```python
from build123d import *

# Parameters (mm, degrees)
BOSS_EXTRUDE1_DEPTH      = 80
F_6_0_6_DIAMETER_HOLE1_D = 6
F_8_0_8_DIAMETER_HOLE1_D = 8
F_6_0_6_DIAMETER_HOLE2_D = 6


with BuildPart() as part:
    # Sketch2 → Boss-Extrude1 (new body)
    with BuildSketch(Plane.XY):
        Polygon((0, 0), (31.153008197, 0), (31.153008197, 120), (0, 120), (0, 110.293748295), (20, 110.293748295), (20, 9.706251705), (0, 9.706251705), align=None)
    extrude(amount=BOSS_EXTRUDE1_DEPTH)

    # Ø6.0 (6) Diameter Hole1 (through all)
    with Locations(Plane(origin=(0, 120, 0), x_dir=(1, 0, 0), z_dir=(0, 1, 0))):
        with Locations((10, -15)):
            Hole(F_6_0_6_DIAMETER_HOLE1_D / 2)

    # Ø8.0 (8) Diameter Hole1 (through all)
    with Locations(Plane(origin=(31.153008197, 0, 0), x_dir=(0, 0, -1), z_dir=(1, 0, 0))):
        with Locations((-45, 30)):
            Hole(F_8_0_8_DIAMETER_HOLE1_D / 2)

    # Ø6.0 (6) Diameter Hole2 (through all)
    with Locations(Plane(origin=(0, 120, 0), x_dir=(1, 0, 0), z_dir=(0, 1, 0))):
        with Locations((11.153008197, -65)):
            Hole(F_6_0_6_DIAMETER_HOLE2_D / 2)


solid = part.part
```
Source: CAD feature listing. Evaluate the final solid. Frame: model axes, mm. A direction names the side the tool comes from. Give positions to 0.01 mm unless a question says otherwise; leave off trailing zeros. Write each loop counter-clockwise with the first axis right and the second up, starting at its lowest first coordinate (ties: lowest second). Pieces come first, ordered by that corner, then holes.
1. Section query C-C (y = 28). Return the cut outline in (x, z).
2. Material intervals for line 1 along Y through (x, z) = (15.5, 6); line 2 along Z through (x, y) = (10, 4.75); line 3 along X through (y, z) = (7, 65), sorted ascending.
3. Access query for faces 4 (the face through (15, 0, 39)), 5 (the face through (20, 61, 39)). Directions: +Z, -Z, +X, -X, +Y, -Y. A direction counts if a zero-diameter tool reaches every point of the face in a straight line with its end or side. Return the directions, or none.
4. Section query D-D (z = 45). Return the cut outline in (x, y).
5. Section query A-A (z = 65). Return the cut outline in (x, y).
6. First-contact query: pin 1 (12 mm diameter, centred on y = 74.5, z = 42, fed in from -X); pin 2 (6.5 mm diameter, centred on y = 30, z = 45, fed in from +X). Flat tips, straight axial feed; report the tip coordinate or a pass-through.
7. Section query B-B (x = 16). Return the cut outline in (y, z), then the cut area to 3 significant figures.
8. Pull-direction query (Z, two-part tool) for faces 1 (the face through (22, 61, 0)), 2 (the face through (10.65, 4.79, 17.93)), 3 (the face through (16, 120, 39)); classes: +Z half, -Z half, draft (parallel to the pull), parting line (faces both ways), or undercut.
Output values:
1. outline: (20, 0) - (31.15, 0) - (31.15, 41.54) - (20, 41.54) - close; (20, 48.46) - (31.15, 48.46) - (31.15, 80) - (20, 80) - close
2. line 1: y = 0 to 9.71, 110.29 to 120
2. line 2: z = 0 to 12, 18 to 62.23, 67.77 to 80
2. line 3: x = 0 to 8.15, 14.15 to 31.15
3. face 4: +Z, -Z, +X, -X, -Y
3. face 5: +Z, -Z, -X
4. outline: (0, 0) - (31.15, 0) - (31.15, 26) - (20, 26) - (20, 9.71) - (0, 9.71) - close; (0, 110.29) - (20, 110.29) - (20, 34) - (31.15, 34) - (31.15, 120) - (0, 120) - close
5. outline: (0, 0) - (8.15, 0) - (8.15, 9.71) - (0, 9.71) - close; (0, 110.29) - (8.15, 110.29) - (8.15, 120) - (0, 120) - close; (14.15, 0) - (31.15, 0) - (31.15, 120) - (14.15, 120) - (14.15, 110.29) - (20, 110.29) - (20, 9.71) - (14.15, 9.71) - close
6. pin 1: stops at x = 20
6. pin 2: passes through
7. outline: (0, 0) - (9.71, 0) - (9.71, 80) - (0, 80) - close; (110.29, 0) - (120, 0) - (120, 80) - (110.29, 80) - close
7. area: 1,550 mm2
8. face 1: -Z half
8. face 2: undercut
8. face 3: draft
